Design review of the part shown in the three views and the two pictorial views. Dimensions are in mm from the part's minimum x, y and z. A direction names the side the tool comes from. Coordinates: 2 decimals unless noted, no trailing zeros. Write each loop counter-clockwise with the first axis right and the second up, starting at its lowest first coordinate (ties: lowest second). Pieces come first, ordered by that corner, then holes.
Q1. For pin 1 Ø12 at (y, z) = (25.5, 21.5) entering from +X; pin 2 Ø2.5 at (x, z) = (3.2, 3.2) entering from -Y; pin 3 Ø3 at (x, z) = (38, 16.5) entering from +Y; pin 4 Ø1.5 at (x, y) = (32.5, 23.5) entering from +Z, all flat-tipped, find the tip position at first contact; note any pin that passes through.
Q2. Take a section at B-B, the plane z = 40.1. Write out the cut boundary in (x, y), plus the area to 4 significant figures.
Q3. For the marked faces 1, 2, 3 and 4, list the 3-axis set-ups (+Z, -Z, +X, -X, +Y, -Y) from which the entire face can be reached by the end or side of a thin tool; tool diameter is ignored.
Q4. Take a section at D-D, the plane z = 10. Write out the cut boundary in (x, y).
Q5. Take a section at A-A, the plane x = 3.2. Write out the cut boundary in (y, z), plus the area to 4 significant figures.
Q6. Take a section at C-C, the plane y = 7. Write out the cut boundary in (x, z), plus the area to 3 significant figures.
Q7. The part is to be moulded in two halves that separate along Z. For the marked faces 5, 6, 7 and 8, say which applies: released by +Z, released by -Z, zero draft, split by the parting line, or undercut.
Q8. For L1, parallel to Z at x = 40.1, y = 3.25; L2, parallel to Z at x = 13.5, y = 5.25, list the stretches that pass through material, from the lowest coordinate up.
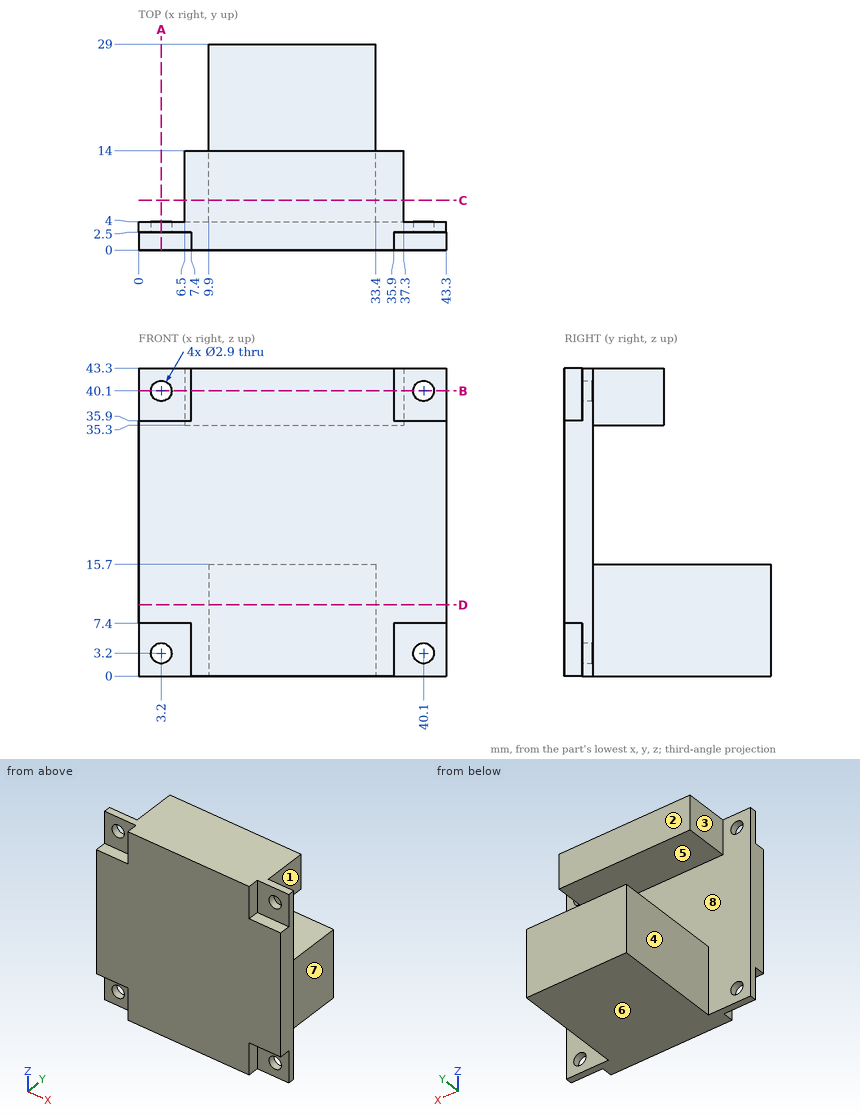
Responses:
1. pin 1: stops at x = 33.4
1. pin 2: passes through
1. pin 3: stops at y = 4
1. pin 4: stops at z = 15.7
2. outline: (0, 2.5) - (1.75, 2.5) - (1.75, 4) - (0, 4) - close; (4.65, 2.5) - (7.4, 2.5) - (7.4, 0) - (35.9, 0) - (35.9, 2.5) - (38.65, 2.5) - (38.65, 4) - (37.3, 4) - (37.3, 14) - (6.5, 14) - (6.5, 4) - (4.65, 4) - close; (41.55, 2.5) - (43.3, 2.5) - (43.3, 4) - (41.55, 4) - close
2. area: 435.5 mm2
3. face 1: +Z, -Z, +X, +Y
3. face 2: +Z, +X, -X, +Y
3. face 3: +Z, -Z, -X, +Y
3. face 4: -Z, -X, +Y
4. outline: (0, 0) - (43.3, 0) - (43.3, 4) - (33.4, 4) - (33.4, 29) - (9.9, 29) - (9.9, 4) - (0, 4) - close
5. outline: (0, 7.4) - (2.5, 7.4) - (2.5, 4.65) - (4, 4.65) - (4, 38.65) - (2.5, 38.65) - (2.5, 35.9) - (0, 35.9) - close; (2.5, 0) - (4, 0) - (4, 1.75) - (2.5, 1.75) - close; (2.5, 41.55) - (4, 41.55) - (4, 43.3) - (2.5, 43.3) - close
5. area: 127.5 mm2
6. outline: (6.5, 35.3) - (37.3, 35.3) - (37.3, 43.3) - (6.5, 43.3) - close; (9.9, 0) - (33.4, 0) - (33.4, 15.7) - (9.9, 15.7) - close
6. area: 615 mm2
7. face 5: undercut
7. face 6: released by -Z
7. face 7: zero draft
7. face 8: undercut
8. L1: z = 0 to 1.75, 4.65 to 38.65, 41.55 to 43.3
8. L2: z = 0 to 15.7, 35.3 to 43.3
